```python
from build123d import *

# Parameters (mm, degrees)
F0_W            = 42.3
F0_H            = 42.3
F0_R            = 1.75
F0_R_2          = 2.95
F0_R_3          = 1.5
F0_R_4          = 11.5
F1_DEPTH        = 10
F2_R            = 3
F3_DEPTH        = 3.5
F4_R            = 4.025
F5_DEPTH        = 8
F6_R            = 5.65
F8_DEPTH        = 10
F8_COPIES_COUNT = 12


# Not quite as in the source:
# - a pattern or mirror of a feature is missing from the dataset's text; its kind, count and spacing are read off the source's solid


with BuildPart() as f1:
    # F0 (on Front) → F1 (new body)
    with BuildSketch(Plane.XZ):
        Rectangle(F0_W, F0_H)
        with Locations((-15.5, -15.5)):
            Circle(F0_R, mode=Mode.SUBTRACT)
        with Locations((0, -15.875)):
            Circle(F0_R_2, mode=Mode.SUBTRACT)
        with Locations((15.5, -15.5)):
            Circle(F0_R, mode=Mode.SUBTRACT)
        with Locations((-18, 0)):
            Circle(F0_R_3, mode=Mode.SUBTRACT)
        with Locations((-15.5, 15.5)):
            Circle(F0_R, mode=Mode.SUBTRACT)
        Circle(F0_R_4, mode=Mode.SUBTRACT)
        with Locations((18, 0)):
            Circle(F0_R_3, mode=Mode.SUBTRACT)
        with Locations((0, 15.875)):
            Circle(F0_R_2, mode=Mode.SUBTRACT)
        with Locations((15.5, 15.5)):
            Circle(F0_R, mode=Mode.SUBTRACT)
    extrude(amount=F1_DEPTH)

    # F2 (on face) → F3 (cut)
    with BuildSketch(Plane(origin=(0, 0, 0), x_dir=(-1, 0, 0), z_dir=(0, 1, 0))):
        with Locations((-15.5, 15.5)):
            Circle(F2_R)
        with Locations((15.5, 15.5)):
            Circle(F2_R)
        with Locations((15.5, -15.5)):
            Circle(F2_R)
        with Locations((-15.5, -15.5)):
            Circle(F2_R)
    extrude(amount=-F3_DEPTH, mode=Mode.SUBTRACT)

    # F4 (on face) → F5 (cut)
    with BuildSketch(Plane(origin=(0, 0, 0), x_dir=(-1, 0, 0), z_dir=(0, 1, 0))):
        with Locations((0, 15.875)):
            Circle(F4_R)
        with Locations((0, -15.875)):
            Circle(F4_R)
    extrude(amount=-F5_DEPTH, mode=Mode.SUBTRACT)

    # F6
    f6_edges = [f1.edges().sort_by_distance(p)[0] for p in [
        (21.15, -5, 21.15),
        (21.15, -5, -21.15),
        (-21.15, -5, 21.15),
        (-21.15, -5, -21.15),
    ]]
    fillet(f6_edges, radius=F6_R)

    # F7 (on face) → F8 (join)
    with BuildSketch(Plane(origin=(0, 0, 0), x_dir=(-1, 0, 0), z_dir=(0, 1, 0))):
        with BuildLine():
            ThreePointArc((11.4891304348, -0.4998818386), (11.5, 0), (11.4891304348, 0.4998818386))
            ThreePointArc((11.4891304348, 0.4998818386), (11, 0), (11.4891304348, -0.4998818386))
        make_face()
    f8 = extrude(amount=-F8_DEPTH)

    # F8_copies: F8 ×12 about axis
    f8_copies_axis = Axis((0, 0, 0), (0, 1, 0))
    for i in range(1, F8_COPIES_COUNT):
        add(f8.rotate(f8_copies_axis, i * 360 / F8_COPIES_COUNT))


solid = f1.part
```
Model file for the job. Use its own axes, mm. A direction names the side the tool comes from. Coordinates: 2 decimals unless noted, no trailing zeros. Loops run counter-clockwise (first coordinate to the right, second up) from the corner with the lowest first, then second, coordinate; pieces in that order, holes last. Notation, with made-up numbers: (37.25, -4.75) -> (87.25, -4.75) arc R33 cw to (87.25, 23.25) -> close; hole circle Ø11 at (40, 42.25). An arc over 180 degrees is marked (long way). Answer as a JSON object with one key per item and string values.
Q1. Cut at A-A (x = 0). List the corners of the cut face in (y, z) (3 decimals), and give its area (3 significant figures).
Report:
{"outline": "(-10, -21.15) -> (0, -21.15) -> (0, -19.9) -> (-8, -19.9) -> (-8, -18.825) -> (-10, -18.825) -> close; (-10, -12.925) -> (-8, -12.925) -> (-8, -11.85) -> (0, -11.85) -> (0, -11) -> (-10, -11) -> close; (-10, 11) -> (0, 11) -> (0, 11.85) -> (-8, 11.85) -> (-8, 12.925) -> (-10, 12.925) -> close; (-10, 18.825) -> (-8, 18.825) -> (-8, 19.9) -> (0, 19.9) -> (0, 21.15) -> (-10, 21.15) -> close", "area": "50.6 mm2"}
Q2. 3-axis set-ups, long thin cutter, end or side, ignore diameter. For faces 1 (the cylindrical face through (19.45, -5.07, -19.54)), 2 (the cylindrical face through (11.117, -4.93, 2.942)): which of +Z, -Z, +X, -X, +Y, -Y reach the whole face in a straight line?
Report:
{"face 1": "-Z, +X, +Y, -Y", "face 2": "+Y, -Y"}
Q3. Cut at B-B (z = 0). List the corners of the cut face in (x, y).
Report:
{"outline": "(-21.15, -10) -> (-19.5, -10) -> (-19.5, 0) -> (-21.15, 0) -> close; (-16.5, -10) -> (-11, -10) -> (-11, 0) -> (-16.5, 0) -> close; (11, -10) -> (16.5, -10) -> (16.5, 0) -> (11, 0) -> close; (19.5, -10) -> (21.15, -10) -> (21.15, 0) -> (19.5, 0) -> close"}
Q4. Cut at C-C (x = 7). List the corners of the cut face in (y, z).
Report:
{"outline": "(-10, -21.15) -> (0, -21.15) -> (0, -9.12) -> (-10, -9.12) -> close; (-10, 9.12) -> (0, 9.12) -> (0, 21.15) -> (-10, 21.15) -> close"}
Q5. Cut at D-D (z = -16.5). List the corners of the cut face in (x, y), and give its area (3 significant figures).
Report:
{"outline": "(-21.06, -10) -> (-16.94, -10) -> (-16.94, -3.5) -> (-18.33, -3.5) -> (-18.33, 0) -> (-21.06, 0) -> close; (-14.06, -10) -> (-2.88, -10) -> (-2.88, -8) -> (-3.98, -8) -> (-3.98, 0) -> (-12.67, 0) -> (-12.67, -3.5) -> (-14.06, -3.5) -> close; (2.88, -10) -> (14.06, -10) -> (14.06, -3.5) -> (12.67, -3.5) -> (12.67, 0) -> (3.98, 0) -> (3.98, -8) -> (2.88, -8) -> close; (16.94, -10) -> (21.06, -10) -> (21.06, 0) -> (18.33, 0) -> (18.33, -3.5) -> (16.94, -3.5) -> close", "area": "269 mm2"}
Q6. Probe probe 1 along Z at (x, y) = (15.5, -6); probe 2 along Z at (x, y) = (15.5, -1.9); probe 3 along Z at (x, y) = (-18, -3.25). List the from-to ranges inside material, lowest first.
Report:
{"probe 1": "z = -21.15 to -17.25, -13.75 to 13.75, 17.25 to 21.15", "probe 2": "z = -21.15 to -18.5, -12.5 to 12.5, 18.5 to 21.15", "probe 3": "z = -20.57 to -17.16, -13.84 to -1.5, 1.5 to 13.84, 17.16 to 20.57"}
Q7. Flat gauge pins, fed straight in: P1, Ø7, axis at x = -15.5, z = 15.5, coming from the -Y side; P2, Ø1.8, axis at x = -16.5, z = 16, coming from the +Y side; P3, Ø4.5, axis at x = 0, z = 15.875, coming from the +Y side. Where does each tip first touch, or does it go through?
Report:
{"P1": "stops at y = -10", "P2": "stops at y = -3.5", "P3": "passes through"}
Q8. Pull direction Z, two halves, no side cores. Call faces 3 (the cylindrical face through (-11.1, -4.9, 3)), 4 (the flat face through (0, -5, 21.15)), 5 (the flat face through (0, -5, -21.15)): released by +Z, released by -Z, zero draft, split by the parting line, or undercut.
Report:
{"face 3": "undercut", "face 4": "released by +Z", "face 5": "released by -Z"}
